```python
from build123d import *

# Parameters (mm, degrees)
SKETCH2_W           = 24
SKETCH2_H           = 47
BOSS_EXTRUDE1_DEPTH = 6
SKETCH3_W           = 24
SKETCH3_H           = 7
BOSS_EXTRUDE2_DEPTH = 10
HOLE1_OUTLINE_R     = 2.15
HOLE1_DEPTH         = 6
HOLE1_START         = 6
HOLE1_2_OUTLINE_R   = 1.7
HOLE1_2_DEPTH       = 1
FILLET1_R           = 4
FILLET2_R           = 0.8


# Read off the part's stored shape, not the designer's step: Hole1, CBORE for M3 SBHCS1
with BuildPart() as part:
    # Sketch2 → Boss-Extrude1 (new body)
    with BuildSketch(Plane.XY):
        with Locations((12, -16.5)):
            Rectangle(SKETCH2_W, SKETCH2_H)
    extrude(amount=BOSS_EXTRUDE1_DEPTH)

    # Sketch3 → Boss-Extrude2 (add)
    with BuildSketch(Plane(origin=(0, 0, 0), x_dir=(-1, 0, 0), z_dir=(0, 0, -1))):
        with Locations((-12, 3.5)):
            Rectangle(SKETCH3_W, SKETCH3_H)
    extrude(amount=BOSS_EXTRUDE2_DEPTH)

    # Hole1 outline → Hole1 (cut)
    with BuildSketch(Plane(origin=(0, 0, 0), x_dir=(1, 0, 0), z_dir=(0, 1, 0))):
        with Locations((3, 5)):
            Circle(HOLE1_OUTLINE_R)
        with Locations((21, 5)):
            Circle(HOLE1_OUTLINE_R)
    extrude(amount=HOLE1_DEPTH, mode=Mode.SUBTRACT)

    # Hole1 2 outline → Hole1 2 (cut)
    with BuildSketch(Plane(origin=(0, 0, 0), x_dir=(1, 0, 0), z_dir=(0, 1, 0)).offset(HOLE1_START)):
        with Locations((3, 5)):
            Circle(HOLE1_2_OUTLINE_R)
        with Locations((21, 5)):
            Circle(HOLE1_2_OUTLINE_R)
    extrude(amount=HOLE1_2_DEPTH, mode=Mode.SUBTRACT)

    # CBORE for M3 SBHCS1 outline → CBORE for M3 SBHCS1 (revolve, cut)
    with BuildSketch(Plane(origin=(18, -30, 0), x_dir=(1, 0, 0), z_dir=(0, -1, 0))):
        Polygon((1.7, 1.65), (1.7, 6), (0, 6), (0, 0), (3.375, 0), (3.35, 0.025), (3.35, 1.65), align=None)
    revolve(axis=Axis((18, -30, 0), (0, 0, 1)), mode=Mode.SUBTRACT)

    # CBORE for M3 SBHCS1 2 outline → CBORE for M3 SBHCS1 2 (revolve, cut)
    with BuildSketch(Plane(origin=(6, -30, 0), x_dir=(1, 0, 0), z_dir=(0, -1, 0))):
        Polygon((0, 0), (3.375, 0), (3.35, 0.025), (3.35, 1.65), (1.7, 1.65), (1.7, 6), (0, 6), align=None)
    revolve(axis=Axis((6, -30, 0), (0, 0, 1)), mode=Mode.SUBTRACT)

    # Fillet1
    fillet1_edges = [part.edges().sort_by_distance(p)[0] for p in [
        (12, 7, 6),
    ]]
    fillet(fillet1_edges, radius=FILLET1_R)

    # Fillet2
    fillet2_edges = [part.edges().sort_by_distance(p)[0] for p in [
        (24, -40, 3),
        (0, -40, 3),
        (12, -40, 6),
        (24, -18.5, 6),
        (12, 0, 0),
        (24, 0, -5),
        (0, 0, -5),
        (24, 3.5, -10),
        (12, 0, -10),
        (0, 3.5, -10),
        (12, 7, -10),
        (0, -18.5, 6),
        (24, 7, -4),
        (0, 7, -4),
        (24, 5.828427125, 4.828427125),
        (24, -20, 0),
        (0, 5.828427125, 4.828427125),
        (12, -40, 0),
        (0, -20, 0),
    ]]
    fillet(fillet2_edges, radius=FILLET2_R)


solid = part.part
```
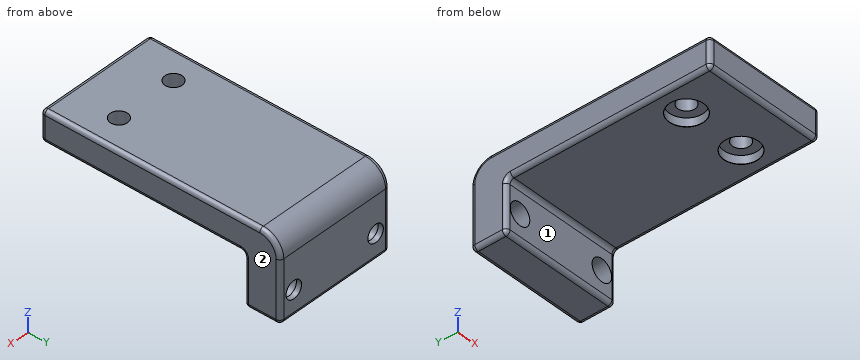
The listing builds one solid part. Answer for the finished solid, in the listing's coordinates (mm). Face numbers are marked on the shaded views. A direction names the side the tool comes from. Give positions to 0.01 mm unless a question says otherwise; leave off trailing zeros. Order: outer loops, then holes, each group sorted by start corner. A loop starts at its lowest first (then second) coordinate and runs counter-clockwise, first axis right, second up. Notation, with made-up numbers: (71.5, 81) -> (92.5, 81) arc R27 ccw to (92.5, 105) -> close; hole circle Ø1 at (32.25, -27). An arc over 180 degrees is marked (long way). Answer as a JSON object with one key per item and string values. Group by question number.
Item 1: The part is cut by section A-A on x = 18. Write down the section's boundary in (y, z) (3 decimals).
Item 2: The part is cut by section C-C on y = 2. Write down the section's boundary in (x, z), and give its area (3 significant figures).
Item 3: The part is cut by section D-D on z = -1.75. Write down the section's boundary in (x, y).
Item 4: Consider L1, parallel to X at y = 4.75, z = -5; L2, parallel to Y at x = 6, z = 0.9; L3, parallel to X at y = 6.6, z = -5. Determine where each line is inside the solid, lowest interval first. Write a range as from..to.
Item 5: A tool of negligible diameter and unlimited length cuts with its end or side. For the marked faces 1 and 2, from which of +Z, -Z, +X, -X, +Y, -Y can it reach the whole face along a straight path? Write none if from no direction.
Item 6: The part is cut by section B-B on z = -5. Write down the section's boundary in (x, y), and give its area (3 significant figures).
Item 7: Flat-ended cylindrical pins translate along their axes: pin 1 (4 mm diameter, centred on x = 7.5, y = -32, fed in from -Z); pin 2 (3.5 mm diameter, centred on x = 16.5, y = -30, fed in from -Z); pin 3 (4 mm diameter, centred on x = 3, z = -5, fed in from -Y). Find the tip coordinate at first contact, or state that the pin passes through.
Result set:
{
 "1": {"outline": "(-40, 0.8) arc R0.8 ccw to (-39.2, 0) -> (-33.375, 0) -> (-33.35, 0.025) -> (-33.35, 1.65) -> (-31.7, 1.65) -> (-31.7, 6) -> (-39.2, 6) arc R0.8 ccw to (-40, 5.2) -> close; (-28.3, 1.65) -> (-26.65, 1.65) -> (-26.65, 0.025) -> (-26.625, 0) -> (-0.8, 0) arc R0.8 cw to (0, -0.8) -> (0, -9.2) arc R0.8 ccw to (0.8, -10) -> (6.2, -10) arc R0.8 ccw to (7, -9.2) -> (7, 2) arc R4 ccw to (3, 6) -> (-28.3, 6) -> close"},
 "2": {"outline": "(0, -9.2) arc R0.8 ccw to (0.8, -10) -> (23.2, -10) arc R0.8 ccw to (24, -9.2) -> (24, 5.2) arc R0.8 ccw to (23.2, 6) -> (0.8, 6) arc R0.8 ccw to (0, 5.2) -> close; hole circle Ø4.3 at (3, -5); hole circle Ø4.3 at (21, -5)", "area": "354 mm²"},
 "3": {"outline": "(0, 0.8) arc R0.8 ccw to (0.8, 0) -> (23.2, 0) arc R0.8 ccw to (24, 0.8) -> (24, 6.2) arc R0.8 ccw to (23.2, 7) -> (0.8, 7) arc R0.8 ccw to (0, 6.2) -> close"},
 "4": {"L1": "0..0.85, 5.15..18.85, 23.15..24", "L2": "-40..-33.35, -26.65..7", "L3": "0.11..1.3, 4.7..19.3, 22.7..23.89"},
 "5": {"face 1": "-Z, +X, -X, -Y", "face 2": "+Z, -Z, +X, +Y, -Y"},
 "6": {"outline": "(0, 0.8) arc R0.8 ccw to (0.8, 0) -> (0.85, 0) -> (0.85, 6) -> (1.3, 6) -> (1.3, 7) -> (0.8, 7) arc R0.8 ccw to (0, 6.2) -> close; (4.7, 6) -> (5.15, 6) -> (5.15, 0) -> (18.85, 0) -> (18.85, 6) -> (19.3, 6) -> (19.3, 7) -> (4.7, 7) -> close; (22.7, 6) -> (23.15, 6) -> (23.15, 0) -> (23.2, 0) arc R0.8 ccw to (24, 0.8) -> (24, 6.2) arc R0.8 ccw to (23.2, 7) -> (22.7, 7) -> close", "area": "109 mm²"},
 "7": {"pin 1": "z = 0", "pin 2": "z = 1.65", "pin 3": "y = 6"}
}
